Answer from the drawing. Dimensions are ordinates in mm from the lowest x, y and z of the part. A direction names the side the tool comes from. Give positions to 0.01 mm unless a question says otherwise; leave off trailing zeros. Order: outer loops, then holes, each group sorted by start corner. A loop starts at its lowest first (then second) coordinate and runs counter-clockwise, first axis right, second up.
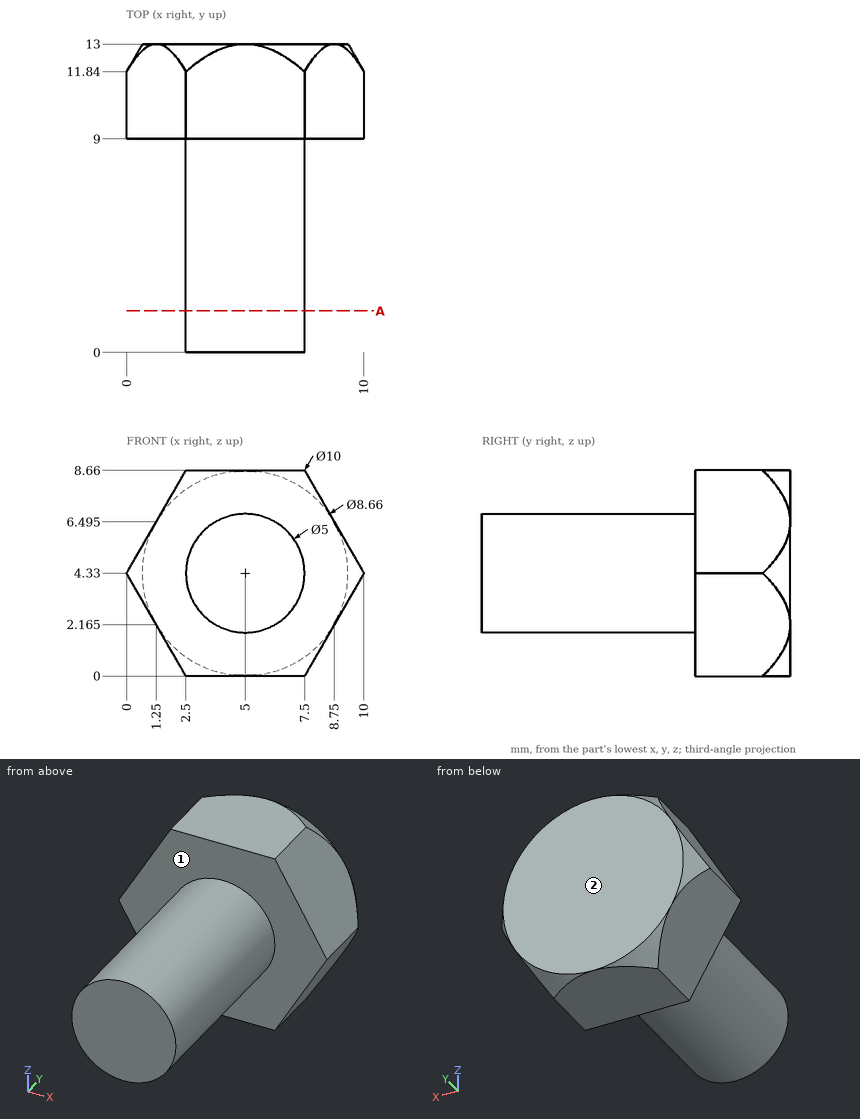
1. Which of the six approach directions +Z, -Z, +X, -X, +Y, -Y give full straight-line access (tool end or side, diameter ignored) to the marked faces 1 and 2?
Findings below:
face 1: -Y
face 2: +Z, -Z, +X, -X, +Y
2. Given P1, Ø5, axis at x = 2, y = 4, coming from the +Z side; P2, Ø2.5, axis at x = 4.5, z = 6.5, coming from the -Y side; P3, Ø2, axis at y = 3, z = 2, coming from the +X side; P4, Ø1.5, axis at x = 1.5, z = 2.5, coming from the -Y side, each flat-ended and moving along its own axis, determine where each tip first touches the part or whether it passes through.
Findings below:
P1: stops at z = 6.78
P2: stops at y = 0
P3: stops at x = 7.12
P4: stops at y = 9
3. Straight lines are drawn through the part: probe 1 along Y at (x, z) = (5.5, 7); probe 2 along Z at (x, y) = (1.25, 10) (1 decimal); probe 3 along Z at (x, y) = (6, 3.25). For each, find the intervals that lie inside material, in ascending order.
Findings below:
probe 1: y = 9 to 13
probe 2: z = 2.2 to 6.5
probe 3: z = 2.04 to 6.62
4. The part is cut by section A-A (y = 1.75). Write down the section's boundary in (x, z).
Findings below:
outline: circle Ø5 at (5, 4.33)
